```python
from build123d import *

# Parameters (mm, degrees)
SKETCH_1_R      = 35
EXTRUDE_1_DEPTH = 5
SKETCH_2_R      = 2.5
EXTRUDE_2_DEPTH = 19
SKETCH_3_R      = 5
EXTRUDE_3_DEPTH = 9
FILLET_1_R      = 5
FILLET_2_R      = 2


with BuildPart() as part:
    # 草图1 → 凸台-拉伸1 (new body)
    with BuildSketch(Plane(origin=(0, 0, 0), x_dir=(1, 0, 0), z_dir=(0, 1, 0))):
        with Locations(Location((0, 0, 0), (0, 0, 270))):
            Circle(SKETCH_1_R)
    extrude(amount=EXTRUDE_1_DEPTH)

    # 草图2 → 凸台-拉伸2 (add)
    with BuildSketch(Plane(origin=(0, 5, 0), x_dir=(1, 0, 0), z_dir=(0, 1, 0))):
        with Locations(Location((0, 0, 0), (0, 0, 270))):
            Circle(SKETCH_2_R)
    extrude(amount=EXTRUDE_2_DEPTH)

    # 草图3 → 凸台-拉伸3 (add)
    with BuildSketch(Plane(origin=(0, 24, 0), x_dir=(1, 0, 0), z_dir=(0, 1, 0))):
        with Locations(Location((0, 0, 0), (0, 0, 270))):
            Circle(SKETCH_3_R)
    extrude(amount=EXTRUDE_3_DEPTH)

    # 圆角1
    fillet_1_edges = [part.edges().sort_by_distance(p)[0] for p in [
        (0, 5, -2.5),
    ]]
    fillet(fillet_1_edges, radius=FILLET_1_R)

    # 圆角2
    fillet_2_edges = [part.edges().sort_by_distance(p)[0] for p in [
        (0, 24, -2.5),
    ]]
    fillet(fillet_2_edges, radius=FILLET_2_R)


solid = part.part
```
Geometry: final body of the model. Coordinates: model frame, mm. A direction names the side the tool comes from. Round coordinates to 2 decimals unless told otherwise and drop trailing zeros. Order: outer loops, then holes, each group sorted by start corner. A loop starts at its lowest first (then second) coordinate and runs counter-clockwise, first axis right, second up. Notation, with made-up numbers: M 3.25,62 L 7.25,62 A11 ccw 7.25,67 Z; hole C 31.25,55 d9. An arc over 180 degrees is marked long. Use one line per item in the form item = value. Start each with the question number.
Q1. Cut plane A-A (x = 0). Return loops of the section in (y, z), and give its area (3 significant figures).
Q2. Access query for faces 1 (the face through (0, 33, 0)), 2 (the face through (-4.88, 28.44, -1.08)). Directions: +Z, -Z, +X, -X, +Y, -Y. A direction counts if a zero-diameter tool reaches every point of the face in a straight line with its end or side. Return the directions, or none.
Q3. Material intervals for line 1 (Y direction, x = 7, z = 30.5); line 2 (X direction, y = 4.5, z = 16.5); line 3 (Z direction, x = -3, y = 26), sorted ascending. Write a range as [from, to].
Q4. Pin query (flat end, axial travel): pin 1 Ø8 at (x, z) = (17, -19) entering from +Y; pin 2 Ø10 at (x, y) = (-3, 28.5) entering from -Z; pin 3 Ø12 at (y, z) = (8, -22.5) entering from +X. Return the tip coordinate at first contact, or that it passes through.
Q5. Cut plane C-C (y = 27). Return loops of the section in (x, z).
Q6. Cut plane B-B (z = 0). Return loops of the section in (x, y), and give its area (3 significant figures).
Q7. Mould query, pull axis Y, two halves, no side actions, for faces 3 (the face through (-2.44, 15.92, -0.54)), 4 (the face through (-21, 2, -28)), 5 (the face through (0, 0, 0)). Classes: +Y half, -Y half, draft (parallel to the pull), parting line (faces both ways), or undercut.
Q8. Cut plane D-D (x = -28). Return loops of the section in (y, z).
Geometry results:
q1.outline = M 0,-35 L 5,-35 L 5,-7.5 A5 cw 10,-2.5 L 22,-2.5 A2 cw 24,-4.5 L 24,-5 L 33,-5 L 33,5 L 24,5 L 24,4.5 A2 cw 22,2.5 L 10,2.5 A5 cw 5,7.5 L 5,35 L 0,35 Z
q1.area = 547 mm^2
q2.face_1 = +Z, -Z, +X, -X, +Y
q2.face_2 = +Y
q3.line_1 = [0, 5]
q3.line_2 = [-30.87, 30.87]
q3.line_3 = [-4, 4]
q4.pin_1 = 5
q4.pin_2 = -5
q4.pin_3 = 30.42
q5.outline = C 0,0 d10
q6.outline = M -35,0 L 35,0 L 35,5 L 7.5,5 A5 cw 2.5,10 L 2.5,22 A2 cw 4.5,24 L 5,24 L 5,33 L -5,33 L -5,24 L -4.5,24 A2 cw -2.5,22 L -2.5,10 A5 cw -7.5,5 L -35,5 Z
q6.area = 547 mm^2
q7.face_3 = undercut
q7.face_4 = draft
q7.face_5 = -Y half
q8.outline = M 0,-21 L 5,-21 L 5,21 L 0,21 Z
